Could you check a few things on this model? Use its own coordinates, in mm. Face numbers are marked on the shaded views. A direction names the side the tool comes from. Round coordinates to 2 decimals unless told otherwise and drop trailing zeros. Write each loop counter-clockwise with the first axis right and the second up, starting at its lowest first coordinate (ties: lowest second). Pieces come first, ordered by that corner, then holes.
```python
from build123d import *

# Parameters (mm, degrees)
SKETCH013_R      = 1.65
EXTRUDE009_DEPTH = 5
SKETCH015_R      = 1.2
EXTRUDE011_DEPTH = 10
SKETCH006_W      = 11.2
SKETCH006_H      = 38
EXTRUDE001_DEPTH = 1
SKETCH007_R      = 1
SKETCH007_W      = 6.4
SKETCH007_H      = 15
EXTRUDE005_DEPTH = 2.6
SKETCH005_W      = 51.25
SKETCH005_H      = 53
EXTRUDE_DEPTH    = 2


with BuildPart() as basecut001:
    # Sketch013 → Extrude009 (new body)
    with BuildSketch(Plane.XY.offset(10.25)):
        with Locations((22.75, 26.5)):
            Circle(SKETCH013_R)
    extrude(amount=-EXTRUDE009_DEPTH)


with BuildPart() as basecuts:
    # Sketch015 → Extrude011 (new body)
    with BuildSketch(Plane.XY):
        with Locations((22.75, 26.5)):
            Circle(SKETCH015_R)
    extrude(amount=EXTRUDE011_DEPTH)

    # Fusion006: union baseCut001
    add(basecut001.part)


with BuildPart() as base002:
    # Sketch006 → Extrude001 (new body)
    with BuildSketch(Plane.XY.offset(2)):
        with Locations((37.6, 27)):
            Rectangle(SKETCH006_W, SKETCH006_H)
    extrude(amount=EXTRUDE001_DEPTH)


with BuildPart() as base003:
    # Sketch007 → Extrude005 (new body)
    with BuildSketch(Plane.XY.offset(2)):
        with Locations((28.675, 48.25)):
            Circle(SKETCH007_R)
        with Locations((46.475, 48.25)):
            Circle(SKETCH007_R)
        with Locations((28.675, 2.55)):
            Circle(SKETCH007_R)
        with Locations((46.475, 2.55)):
            Circle(SKETCH007_R)
        Polygon((3.25, 0), (5.25, 0), (5.25, 5.25), (6.75, 5.25), (6.75, 7.25), (3.25, 7.25), align=None)
        Polygon((17.75, 0), (15.75, 0), (15.75, 1.1), (15.3, 1.1), (15.3, 1.9), (15.75, 1.9), (15.75, 5.25), (14.25, 5.25), (14.25, 7.25), (17.75, 7.25), align=None)
        with Locations((22.7, 27.5)):
            Rectangle(SKETCH007_W, SKETCH007_H)
    extrude(amount=EXTRUDE005_DEPTH)


with BuildPart() as bottom:
    # Sketch005 → Extrude (new body)
    with BuildSketch(Plane.XY):
        with Locations((25.625, 26.5)):
            Rectangle(SKETCH005_W, SKETCH005_H)
    extrude(amount=EXTRUDE_DEPTH)

    # Fusion002: union base002, base003
    add(base002.part)
    add(base003.part)

    # Cut001: cut baseCuts
    add(basecuts.part, mode=Mode.SUBTRACT)


solid = bottom.part
```
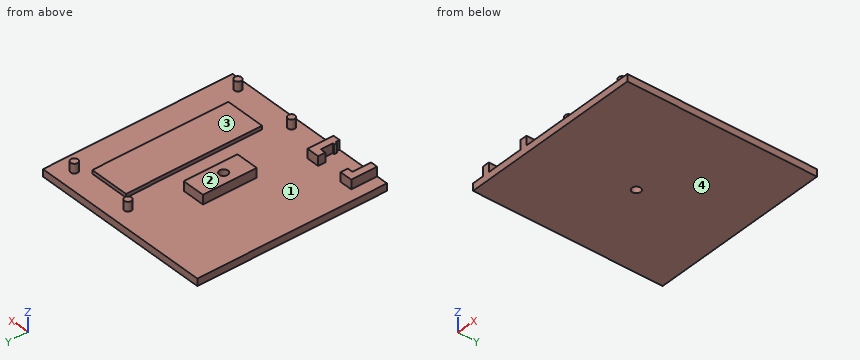
Q1. I'm going to push flat-ended pins straight in: pin 1 Ø1.1 at (x, z) = (37.5, 2.5) entering from -Y; pin 2 Ø0.8 at (x, z) = (35, 2.5) entering from +Y; pin 3 Ø0.8 at (y, z) = (3, 3) entering from +X; pin 4 Ø0.5 at (x, z) = (15.5, 3) entering from +Y. Where does each tip first touch, or does it pass through?
Q2. If I drill on L1, parallel to Y at x = 22.75, z = 2.5; L2, parallel to X at y = 26.5, z = 1.5; L3, parallel to Y at x = 22.75, z = 1.4, over which ranges is the centre line in solid material (lowest first)?
Q3. Imagine slicing it at A-A, the plane z = 3.65. Write out the boundary of the cut face in (x, y) (3 decimals).
Q4. Imagine slicing it at D-D, the plane x = 40. Write out the boundary of the cut face in (y, z).
Q5. On a 3-axis mill with a long thin cutter (end or side, diameter ignored), from which of +Z, -Z, +X, -X, +Y, -Y can I reach the whole of each face in a straight line? I mean the marked faces 3 and 4. Say none if no direction works.
Q6. Imagine slicing it at C-C, the plane y = 2.55. Write out the boundary of the cut face in (x, z) (3 decimals), then the cut area to 3 significant figures.
Q7. We'd pull the mould along X, two halves only. Please class the marked faces 1 and 2: pulls with the +X half, pulls with the -X half, needs draft (parallel to the pull), parting line crosses it, or undercut.
Q8. Imagine slicing it at B-B, the plane x = 22.75. Write out the boundary of the cut face in (y, z), then the cut area to 3 significant figures.
Results found:
1. pin 1: stops at y = 0
1. pin 2: stops at y = 46
1. pin 3: stops at x = 47.47
1. pin 4: stops at y = 7.25
2. L1: y = 20 to 25.3, 27.7 to 35
2. L2: x = 0 to 21.55, 23.95 to 51.25
2. L3: y = 0 to 25.3, 27.7 to 53
3. outline: (3.25, 0) - (5.25, 0) - (5.25, 5.25) - (6.75, 5.25) - (6.75, 7.25) - (3.25, 7.25) - close; (14.25, 5.25) - (15.75, 5.25) - (15.75, 1.9) - (15.3, 1.9) - (15.3, 1.1) - (15.75, 1.1) - (15.75, 0) - (17.75, 0) - (17.75, 7.25) - (14.25, 7.25) - close; (19.5, 20) - (25.9, 20) - (25.9, 35) - (19.5, 35) - close; circle Ø2 at (28.675, 2.55); circle Ø2 at (28.675, 48.25); circle Ø2 at (46.475, 2.55); circle Ø2 at (46.475, 48.25); hole circle Ø2.4 at (22.75, 26.5)
4. outline: (0, 0) - (53, 0) - (53, 2) - (46, 2) - (46, 3) - (8, 3) - (8, 2) - (0, 2) - close
5. face 3: +Z, +X, +Y, -Y
5. face 4: -Z, +X, -X, +Y, -Y
6. outline: (0, 0) - (51.25, 0) - (51.25, 2) - (47.475, 2) - (47.475, 4.6) - (45.475, 4.6) - (45.475, 2) - (29.675, 2) - (29.675, 4.6) - (27.675, 4.6) - (27.675, 2) - (17.75, 2) - (17.75, 4.6) - (15.75, 4.6) - (15.75, 2) - (5.25, 2) - (5.25, 4.6) - (3.25, 4.6) - (3.25, 2) - (0, 2) - close
6. area: 123 mm2
7. face 1: undercut
7. face 2: needs draft
8. outline: (0, 0) - (25.3, 0) - (25.3, 4.6) - (20, 4.6) - (20, 2) - (0, 2) - close; (27.7, 0) - (53, 0) - (53, 2) - (35, 2) - (35, 4.6) - (27.7, 4.6) - close
8. area: 134 mm2
